```python
from build123d import *

# Parameters (mm, degrees)
SKETCH1_R           = 3.4
BOSS_EXTRUDE1_DEPTH = 440


with BuildPart() as part:
    # Sketch1 → Boss-Extrude1 (new body)
    with BuildSketch(Plane.XZ):
        with BuildLine():
            Line((-8.24999678, 13.000000511), (-4.100001047, 13.000000511))
            Line((-4.100001047, 13.000000511), (-4.100001047, 13.9999993))
            Line((-4.100001047, 13.9999993), (-5.100001047, 13.9999993))
            Line((-5.100001047, 13.9999993), (-5.100001047, 15.000001161))
            Line((-5.100001047, 15.000001161), (-12.9999991, 15.000001161))
            ThreePointArc((-12.9999991, 15.000001161), (-14.414213082, 14.414214549), (-14.999999693, 13.000000567))
            Line((-14.999999693, 13.000000567), (-14.999999693, 5.099999792))
            Line((-14.999999693, 5.099999792), (-14.000001367, 5.099999792))
            Line((-14.000001367, 5.099999792), (-14.000001367, 4.099999792))
            Line((-14.000001367, 4.099999792), (-12.999980958, 4.099999792))
            Line((-12.999980958, 4.099999792), (-12.999980958, 8.250012005))
            Line((-12.999980958, 8.250012005), (-9.664201657, 8.250012005))
            Line((-9.664201657, 8.250012005), (-5.514202303, 4.100011174))
            Line((-5.514202303, 4.100011174), (-5.514202303, -4.099988826))
            Line((-5.514202303, -4.099988826), (-9.664194622, -8.249987936))
            Line((-9.664194622, -8.249987936), (-12.999980958, -8.249987936))
            Line((-12.999980958, -8.249987936), (-12.999980958, -4.100000208))
            Line((-12.999980958, -4.100000208), (-14.000001367, -4.100000208))
            Line((-14.000001367, -4.100000208), (-14.000001367, -5.100000208))
            Line((-14.000001367, -5.100000208), (-14.999999693, -5.100000208))
            Line((-14.999999693, -5.100000208), (-14.999999693, -13.000000955))
            ThreePointArc((-14.999999693, -13.000000955), (-14.414213128, -14.414214825), (-12.999999257, -15.000001391))
            Line((-12.999999257, -15.000001391), (-5.100001047, -15.000001391))
            Line((-5.100001047, -15.000001391), (-5.100001047, -14.000000699))
            Line((-5.100001047, -14.000000699), (-4.100001047, -14.000000699))
            Line((-4.100001047, -14.000000699), (-4.100001047, -13.000000927))
            Line((-4.100001047, -13.000000927), (-8.24999678, -13.000000927))
            Line((-8.24999678, -13.000000927), (-8.24999678, -9.664217294))
            Line((-8.24999678, -9.664217294), (-4.09999914, -5.514212907))
            Line((-4.09999914, -5.514212907), (4.100018356, -5.514212907))
            Line((4.100018356, -5.514212907), (8.250001062, -9.66419709))
            Line((8.250001062, -9.66419709), (8.250001062, -13.000000927))
            Line((8.250001062, -13.000000927), (4.099987439, -13.000000927))
            Line((4.099987439, -13.000000927), (4.099987439, -14.000000699))
            Line((4.099987439, -14.000000699), (5.099987459, -14.000000699))
            Line((5.099987459, -14.000000699), (5.099987459, -15.000001391))
            Line((5.099987459, -15.000001391), (12.999985682, -15.000001391))
            ThreePointArc((12.999985682, -15.000001391), (14.414199699, -14.414214765), (14.999986325, -13.000000748))
            Line((14.999986325, -13.000000748), (14.999986325, -5.100000208))
            Line((14.999986325, -5.100000208), (13.999990764, -5.100000208))
            Line((13.999990764, -5.100000208), (13.999990764, -4.100000208))
            Line((13.999990764, -4.100000208), (12.999996372, -4.100000208))
            Line((12.999996372, -4.100000208), (12.999996372, -8.249987936))
            Line((12.999996372, -8.249987936), (9.664201659, -8.249987936))
            Line((9.664201659, -8.249987936), (5.514206692, -4.099991492))
            Line((5.514206692, -4.099991492), (5.514206692, 4.100008559))
            Line((5.514206692, 4.100008559), (9.66420339, 8.250012005))
            Line((9.66420339, 8.250012005), (12.999996372, 8.250012005))
            Line((12.999996372, 8.250012005), (12.999996372, 4.099999792))
            Line((12.999996372, 4.099999792), (13.999990764, 4.099999792))
            Line((13.999990764, 4.099999792), (13.999990764, 5.099999792))
            Line((13.999990764, 5.099999792), (14.999986325, 5.099999792))
            Line((14.999986325, 5.099999792), (14.999986325, 13.000001058))
            ThreePointArc((14.999986325, 13.000001058), (14.414199857, 14.414214693), (12.999986222, 15.000001161))
            Line((12.999986222, 15.000001161), (5.099987459, 15.000001161))
            Line((5.099987459, 15.000001161), (5.099987459, 13.9999993))
            Line((5.099987459, 13.9999993), (4.099987439, 13.9999993))
            Line((4.099987439, 13.9999993), (4.099987439, 13.000000511))
            Line((4.099987439, 13.000000511), (8.250001062, 13.000000511))
            Line((8.250001062, 13.000000511), (8.250001062, 9.664237062))
            Line((8.250001062, 9.664237062), (4.100007893, 5.514237102))
            Line((4.100007893, 5.514237102), (-4.100018481, 5.514237102))
            Line((-4.100018481, 5.514237102), (-8.24999678, 9.664216878))
            Line((-8.24999678, 9.664216878), (-8.24999678, 13.000000511))
        make_face()
        with Locations(Location((-1.0477e-05, -4.16e-07, 0), (0, 0, 90))):
            Circle(SKETCH1_R, mode=Mode.SUBTRACT)
        with BuildLine():
            Line((13.499986967, -10.750000579), (13.499986967, -12.500001267))
            ThreePointArc((13.499986967, -12.500001267), (13.207093572, -13.207108473), (12.499986367, -13.500001867))
            Line((12.499986367, -13.500001867), (10.749986886, -13.500001867))
            ThreePointArc((10.749986886, -13.500001867), (10.042879512, -13.207108403), (9.749986047, -12.500001028))
            Line((9.749986047, -12.500001028), (9.749986047, -10.750001028))
            ThreePointArc((9.749986047, -10.750001028), (10.042879305, -10.042894153), (10.74998618, -9.750000895))
            Line((10.74998618, -9.750000895), (12.499987283, -9.750000895))
            ThreePointArc((12.499987283, -9.750000895), (13.207093841, -10.042894021), (13.499986967, -10.750000579))
        make_face(mode=Mode.SUBTRACT)
        with BuildLine():
            Line((-10.749994869, 9.750000545), (-12.499998542, 9.750000545))
            ThreePointArc((-12.499998542, 9.750000545), (-13.207105378, 10.042893787), (-13.499998619, 10.750000623))
            Line((-13.499998619, 10.750000623), (-13.499998619, 12.500000623))
            ThreePointArc((-13.499998619, 12.500000623), (-13.207105152, 13.207108005), (-12.499997769, 13.500001473))
            Line((-12.499997769, 13.500001473), (-10.749995653, 13.500001473))
            ThreePointArc((-10.749995653, 13.500001473), (-10.04288827, 13.207108005), (-9.749994803, 12.500000623))
            Line((-9.749994803, 12.500000623), (-9.749994803, 10.750000612))
            ThreePointArc((-9.749994803, 10.750000612), (-10.042888041, 10.042893784), (-10.749994869, 9.750000545))
        make_face(mode=Mode.SUBTRACT)
        with BuildLine():
            Line((12.499988487, 9.750000545), (10.74998617, 9.750000545))
            ThreePointArc((10.74998617, 9.750000545), (10.042879302, 10.0428938), (9.749986047, 10.750000668))
            Line((9.749986047, 10.750000668), (9.749986047, 12.500000634))
            ThreePointArc((9.749986047, 12.500000634), (10.042879552, 13.207108106), (10.749987025, 13.500001611))
            Line((10.749987025, 13.500001611), (12.499987646, 13.500001611))
            ThreePointArc((12.499987646, 13.500001611), (13.207095116, 13.207108107), (13.49998862, 12.500000637))
            Line((13.49998862, 12.500000637), (13.49998862, 10.750000679))
            ThreePointArc((13.49998862, 10.750000679), (13.207095362, 10.042893803), (12.499988487, 9.750000545))
        make_face(mode=Mode.SUBTRACT)
        with BuildLine():
            Line((-10.749995791, -13.500002028), (-12.499997631, -13.500002028))
            ThreePointArc((-12.499997631, -13.500002028), (-13.207105111, -13.207108519), (-13.499998619, -12.500001039))
            Line((-13.499998619, -12.500001039), (-13.499998619, -10.750001039))
            ThreePointArc((-13.499998619, -10.750001039), (-13.207105358, -10.042894156), (-12.499998475, -9.750000895))
            Line((-12.499998475, -9.750000895), (-10.749994936, -9.750000895))
            ThreePointArc((-10.749994936, -9.750000895), (-10.042888061, -10.042894153), (-9.749994803, -10.750001028))
            Line((-9.749994803, -10.750001028), (-9.749994803, -12.500001039))
            ThreePointArc((-9.749994803, -12.500001039), (-10.042888311, -13.207108519), (-10.749995791, -13.500002028))
        make_face(mode=Mode.SUBTRACT)
    extrude(amount=-BOSS_EXTRUDE1_DEPTH)


solid = part.part
```
The model under review builds one solid part; all positions refer to its coordinate system, in mm. A direction names the side the tool comes from. Coordinates: 2 decimals unless noted, no trailing zeros. Answer in a Markdown table with one row per item. Add a question column.
Q1. For faces 1 (the face through (0, 217, -5.514)), 2 (the face through (0, 217, 5.514)), 3 (the face through (-5.514, 217, 0)), list the 3-axis set-ups (+Z, -Z, +X, -X, +Y, -Y) from which the entire face can be reached by the end or side of a thin tool; tool diameter is ignored.
Q2. Consider section A-A on y = 393.5. Give the number of separate pieces and of enclosed holes in the cut face, then the cut area to 3 significant figures.
Q3. Draft analysis for pull direction Z (two halves, no side actions). For faces 4 (the face through (9, 217, -15)), 5 (the face through (5.514, 217, 0)), 6 (the face through (9, 217, 15)), 7 (the face through (-4, 440, 0)), state which applies: +Z half, -Z half, draft (parallel to the pull), parting line (faces both ways), or undercut.
Q4. To check wall thickness, follow line 1 along X through (y, z) = (389, -12); line 2 along X through (y, z) = (351, 0). State the ranges of each line that lie inside material, in increasing order. Write a range as from..to.
Q5. Clearance check with flat-ended pins moving along their axes: pin 1 (10 mm diameter, centred on x = 0.5, y = 160.5, fed in from -Z); pin 2 (6.5 mm diameter, centred on x = -0.5, y = 176.5, fed in from -Z); pin 3 (2 mm diameter, centred on x = -1, y = 373.5, fed in from +Z); pin 4 (1.1 mm diameter, centred on y = 203, z = 14.5, fed in from -X). State where each tip first meets the part, or that it passes through.
Answers below:
| question | item | result |
|---|---|---|
| 1 | face 1 | -Z, +Y, -Y |
| 1 | face 2 | +Z, +Y, -Y |
| 1 | face 3 | -X, +Y, -Y |
| 2 | separate pieces | 1 |
| 2 | enclosed holes | 5 |
| 2 | area | 309 mm² |
| 3 | face 4 | -Z half |
| 3 | face 5 | undercut |
| 3 | face 6 | +Z half |
| 3 | face 7 | draft |
| 4 | line 1 | -15..-13.5, -9.75..-8.25, 8.25..9.75, 13.5..15 |
| 4 | line 2 | -5.51..-3.4, 3.4..5.51 |
| 5 | pin 1 | z = -15 |
| 5 | pin 2 | z = -5.51 |
| 5 | pin 3 | z = 5.51 |
| 5 | pin 4 | x = -14.76 |
